For this review, take the finished solid that the model builds, in its own axes (mm). Round coordinates to 2 decimals unless told otherwise and drop trailing zeros. Loops run counter-clockwise (first coordinate to the right, second up) from the corner with the lowest first, then second, coordinate; pieces in that order, holes last.
1. Consider section A-A on z = -1.25. State the section outline as (x, y) points (3 decimals), then the cut area to 3 significant figures.
2. Clearance check with flat-ended pins moving along their axes: pin 1 Ø2 at (x, z) = (-1.5, -3) entering from -Y; pin 2 Ø2.5 at (x, y) = (0, 0) entering from +Z. State where each tip first meets the part, or that it passes through.
3. To check wall thickness, follow line 1 along Y through (x, z) = (0.25, 2); line 2 along Y through (x, z) = (-1.25, 3.75); line 3 along X through (y, z) = (-2.75, -3.5). State the ranges of each line that lie inside material, in increasing order.
from build123d import *

# Parameters (mm, degrees)
EXTRUDE1_DEPTH          = 4.7625
EXTRUDE1_DEPTH_BACK     = 4.7625
SKETCH1_R               = 1.4224
SKETCH8_OUTSIDE_W       = 51.56
SKETCH8_OUTSIDE_H       = 52.542
SKETCH8_OUTSIDE_R       = 3.175
EXTRUDE4_DEPTH          = 11.688642726
EXTRUDE4_DRAFT          = -60
MIRROR1_COPY_1_SKETCH_W = 51.56
MIRROR1_COPY_1_SKETCH_H = 52.542
MIRROR1_COPY_1_SKETCH_R = 3.175
MIRROR1_COPY_1_DEPTH    = 11.688642726
MIRROR1_COPY_1_DRAFT    = -60


with BuildPart() as part:
    # Sketch1 → Extrude1 (new, two sides: drawn at the far end of the back side and taken through both)
    with BuildSketch(Plane.XY.offset(-EXTRUDE1_DEPTH_BACK)):
        Polygon((0, 3.666174209), (-3.175, 1.833087105), (-3.175, -1.833087105), (0, -3.666174209), (3.175, -1.833087105), (3.175, 1.833087105), align=None)
        with Locations(Location((0, 0, 0), (0, 0, 180))):
            Circle(SKETCH1_R, mode=Mode.SUBTRACT)
    extrude(amount=EXTRUDE1_DEPTH + EXTRUDE1_DEPTH_BACK)

    # Extrude3 cone 1 section (through the dimple's axis) → Extrude3 (revolve, cut)
    with BuildSketch(Plane(origin=(0, 0, -4.7625), x_dir=(0, 1, 0), z_dir=(1, 0, 0))):
        Polygon((0, 0), (1.4732, 0), (0, 1.579813584), align=None)
    extrude3 = revolve(axis=Axis((0, 0, -4.7625), (0, 0, 1)), mode=Mode.SUBTRACT)


with BuildPart() as extrude4_tool:
    # Sketch8 outside → Extrude4 (with draft: the straight prism first)
    with BuildSketch(Plane(origin=(0, 0, -4.7625), x_dir=(-1, 0, 0), z_dir=(0, 0, -1))):
        Rectangle(SKETCH8_OUTSIDE_W, SKETCH8_OUTSIDE_H)
        Circle(SKETCH8_OUTSIDE_R, mode=Mode.SUBTRACT)
    extrude(amount=-EXTRUDE4_DEPTH)
    # Extrude4: the draft: its side faces are tilted about the plane it starts from
    extrude4_sides = [extrude4_tool.faces().sort_by_distance(p)[0] for p in [
        (0, -26.271, 1.081821363),
        (-25.78, 0, 1.081821363),
        (0, 26.271, 1.081821363),
        (25.78, 0, 1.081821363),
        (3.175, 0, 1.081821363),
    ]]
    draft(extrude4_sides, Plane(origin=(0, 0, -4.7625), x_dir=(-1, 0, 0), z_dir=(0, 0, -1)), EXTRUDE4_DRAFT)


with BuildPart() as part_1:
    add(part.part)

    # Extrude4: cut by extrude4_tool
    add(extrude4_tool.part, mode=Mode.SUBTRACT)

    # Mirror1: Extrude3 across plane
    add(extrude3.mirror(Plane.XY), mode=Mode.SUBTRACT)


with BuildPart() as mirror1_copy_1_tool:
    # Mirror1 copy 1 sketch → Mirror1 copy 1 (with draft: the straight prism first)
    with BuildSketch(Plane(origin=(0, 0, 4.7625), x_dir=(-1, 0, 0), z_dir=(0, 0, 1))):
        Rectangle(MIRROR1_COPY_1_SKETCH_W, MIRROR1_COPY_1_SKETCH_H)
        Circle(MIRROR1_COPY_1_SKETCH_R, mode=Mode.SUBTRACT)
    extrude(amount=-MIRROR1_COPY_1_DEPTH)
    # Mirror1 copy 1: the draft: its side faces are tilted about the plane it starts from
    mirror1_copy_1_sides = [mirror1_copy_1_tool.faces().sort_by_distance(p)[0] for p in [
        (0, -26.271, -1.081821363),
        (-25.78, 0, -1.081821363),
        (0, 26.271, -1.081821363),
        (25.78, 0, -1.081821363),
        (3.175, 0, -1.081821363),
    ]]
    draft(mirror1_copy_1_sides, Plane(origin=(0, 0, 4.7625), x_dir=(-1, 0, 0), z_dir=(0, 0, 1)), MIRROR1_COPY_1_DRAFT)


with BuildPart() as part_2:
    add(part_1.part)

    # Mirror1 copy 1: cut by mirror1_copy_1_tool
    add(mirror1_copy_1_tool.part, mode=Mode.SUBTRACT)


solid = part_2.part
Resolved:
1. outline: (-3.175, -1.833) - (0, -3.666) - (3.175, -1.833) - (3.175, 1.833) - (0, 3.666) - (-3.175, 1.833) - close; hole circle Ø2.845 at (0, 0)
1. area: 28.6 mm2
2. pin 1: stops at y = -3.38
2. pin 2: passes through
3. line 1: y = -3.52 to -1.4, 1.4 to 3.52
3. line 2: y = -2.94 to -0.68, 0.68 to 2.94
3. line 3: x = -1.59 to 1.59
